from build123d import *

# Parameters (mm, degrees)
SKETCH1_R                = 5.5
SKETCH1_R_2              = 3.9
BOSS_EXTRUDE1_DEPTH      = 14
BOSS_EXTRUDE2_DEPTH      = 30.85
BOSS_EXTRUDE2_DEPTH_BACK = 30.85
SKETCH3_R                = 10
BOSS_EXTRUDE3_DEPTH      = 12.45
SKETCH4_R                = 10
BOSS_EXTRUDE4_DEPTH      = 12.45
CUT_EXTRUDE1_DEPTH       = 3
CUT_EXTRUDE1_DEPTH_BACK  = 3
CUT_EXTRUDE2_DEPTH       = 3
CUT_EXTRUDE2_DEPTH_BACK  = 3


with BuildPart() as part:
    # Sketch1 → Boss-Extrude1 (new body)
    with BuildSketch(Plane(origin=(0, 0, 0), x_dir=(1, 0, 0), z_dir=(0, 1, 0))):
        with BuildLine():
            Line((-18, -44.5), (18, -44.5))
            ThreePointArc((18, -44.5), (24.717514421, -41.717514421), (27.5, -35))
            Line((27.5, -35), (27.5, 35))
            ThreePointArc((27.5, 35), (24.717514421, 41.717514421), (18, 44.5))
            Line((18, 44.5), (-18, 44.5))
            ThreePointArc((-18, 44.5), (-24.717514421, 41.717514421), (-27.5, 35))
            Line((-27.5, 35), (-27.5, -35))
            ThreePointArc((-27.5, -35), (-24.717514421, -41.717514421), (-18, -44.5))
        make_face()
        with Locations((18, 35)):
            Circle(SKETCH1_R, mode=Mode.SUBTRACT)
        with Locations((18, -35)):
            Circle(SKETCH1_R, mode=Mode.SUBTRACT)
        with Locations((0, 35)):
            Circle(SKETCH1_R_2, mode=Mode.SUBTRACT)
        with Locations((0, -35)):
            Circle(SKETCH1_R_2, mode=Mode.SUBTRACT)
        with Locations((-18, 35)):
            Circle(SKETCH1_R, mode=Mode.SUBTRACT)
        with Locations((-18, -35)):
            Circle(SKETCH1_R, mode=Mode.SUBTRACT)
    extrude(amount=BOSS_EXTRUDE1_DEPTH)

    # Sketch2 → Boss-Extrude2 (add, two sides)
    with BuildSketch(Plane.XY) as boss_extrude2_sk:
        Polygon((-28.085675658, 14), (-27.7, 0), (-22.7, 0), (-22.7, 14), align=None)
    extrude(amount=BOSS_EXTRUDE2_DEPTH)
    extrude(boss_extrude2_sk.sketch, amount=-BOSS_EXTRUDE2_DEPTH_BACK)

    # Sketch3 → Boss-Extrude3 (add)
    with BuildSketch(Plane.XY.offset(25)):
        with BuildLine():
            Line((-29.215236642, 55.002986453), (-27.7, 0))
            Line((-27.7, 0), (27.5, 0))
            Line((27.5, 0), (27.5, 16.676103914))
            ThreePointArc((27.5, 16.676103914), (27.466207658, 16.992703195), (27.366353194, 17.295037634))
            Line((27.366353194, 17.295037634), (3.485336194, 70.014582166))
            ThreePointArc((3.485336194, 70.014582166), (-15.37030771, 79.662563606), (-28.994174525, 63.445008121))
            Line((-28.994174525, 63.445008121), (-29.215236642, 55.002986453))
        make_face()
        with Locations((-12, 63)):
            Circle(SKETCH3_R, mode=Mode.SUBTRACT)
    extrude(amount=-BOSS_EXTRUDE3_DEPTH)

    # Sketch4 → Boss-Extrude4 (add)
    with BuildSketch(Plane.XY.offset(-25)):
        with BuildLine():
            Line((-29.215236642, 55.002986453), (-27.7, 0))
            Line((-27.7, 0), (27.5, 0))
            Line((27.5, 0), (27.5, 16.676103914))
            ThreePointArc((27.5, 16.676103914), (27.466207658, 16.992703195), (27.366353194, 17.295037634))
            Line((27.366353194, 17.295037634), (3.485336194, 70.014582166))
            ThreePointArc((3.485336194, 70.014582166), (-15.37030771, 79.662563606), (-28.994174525, 63.445008121))
            Line((-28.994174525, 63.445008121), (-29.215236642, 55.002986453))
        make_face()
        with Locations((-12, 63)):
            Circle(SKETCH4_R, mode=Mode.SUBTRACT)
    extrude(amount=BOSS_EXTRUDE4_DEPTH)

    # Sketch5 → Cut-Extrude1 (cut, two sides)
    with BuildSketch(Plane.XY.offset(25)) as cut_extrude1_sk:
        with BuildLine():
            Line((-9.85, 49.15), (-9.85, 63))
            Line((-9.85, 63), (-14.15, 63))
            Line((-14.15, 63), (-14.15, 49.15))
            ThreePointArc((-14.15, 49.15), (-12, 47), (-9.85, 49.15))
        make_face()
    extrude(amount=CUT_EXTRUDE1_DEPTH, mode=Mode.SUBTRACT)
    extrude(cut_extrude1_sk.sketch, amount=-CUT_EXTRUDE1_DEPTH_BACK, mode=Mode.SUBTRACT)

    # Sketch6 → Cut-Extrude2 (cut, two sides)
    with BuildSketch(Plane.XY.offset(-25)) as cut_extrude2_sk:
        with BuildLine():
            Line((-9.85, 49.15), (-9.85, 63))
            Line((-9.85, 63), (-14.15, 63))
            Line((-14.15, 63), (-14.15, 49.15))
            ThreePointArc((-14.15, 49.15), (-12, 47), (-9.85, 49.15))
        make_face()
    extrude(amount=CUT_EXTRUDE2_DEPTH, mode=Mode.SUBTRACT)
    extrude(cut_extrude2_sk.sketch, amount=-CUT_EXTRUDE2_DEPTH_BACK, mode=Mode.SUBTRACT)


solid = part.part
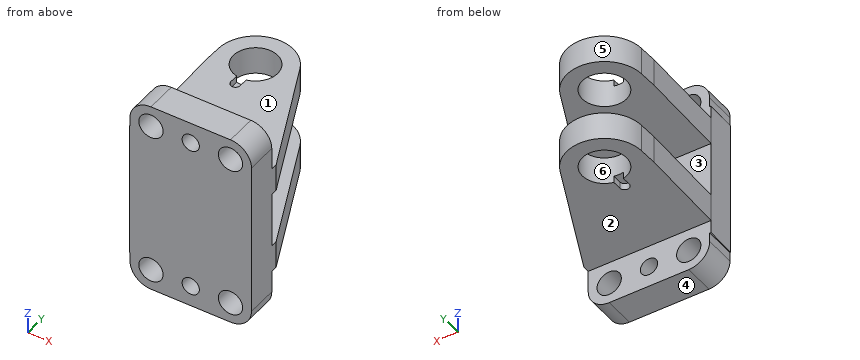
Check sheet for the modelled part. Datum: model origin and axes. Units: mm. Face numbers are marked on the shaded views. A direction names the side the tool comes from. Give positions to 0.01 mm unless a question says otherwise; leave off trailing zeros. Loops run counter-clockwise (first coordinate to the right, second up) from the corner with the lowest first, then second, coordinate; pieces in that order, holes last. Notation, with made-up numbers: M 69.5,25.5 L 94.5,25.5 A18 ccw 94.5,41.5 Z; hole C 82,84 d8. An arc over 180 degrees is marked long. Return JSON: item names as keys, results as strings. Group by question number.
1. Cross-section at C-C on y = 75. Record the boundary of the cut face in (x, z), plus the area to 3 significant figures.
2. Cross-section at B-B on x = 0. Record the boundary of the cut face in (y, z).
3. Cross-section at D-D on z = -8.5. Record the boundary of the cut face in (x, y), plus the area to 4 significant figures.
4. Mould release check, pull along X, two halves, no side actions. Record for the marked faces 4, 5 and 6: released by +X, released by -X, zero draft, split by the parting line, or undercut.
5. Tool access check on the marked faces 1, 2 and 3. Record the directions out of +Z, -Z, +X, -X, +Y, -Y that give a thin tool (end or side, any length) a straight path to the whole face; none if there is none.
6. Thickness scan on L1, parallel to X at y = 5, z = 35; L2, parallel to Z at x = 18, y = 3; L3, parallel to Z at x = 0, y = 10. Record the ranges inside material, lowest first.
7. Go/stop test with flat-tipped pins: pin 1 (3 mm diameter, centred on y = 43.5, z = 23, fed in from -X); pin 2 (4.5 mm diameter, centred on x = -12, y = 51, fed in from -Z); pin 3 (3 mm diameter, centred on y = 62.5, z = -26, fed in from +X); pin 4 (12.5 mm diameter, centred on x = -18, z = 35, fed in from -Y). Record where each tip stops, or that it passes through.
8. Cross-section at A-A on y = 66.5. Record the boundary of the cut face in (x, z).
Return value:
{
 "1": {"outline": "M -24.04,-25 L 0.04,-25 L 0.04,-12.55 L -24.04,-12.55 Z; M -24.04,12.55 L 0.04,12.55 L 0.04,25 L -24.04,25 Z", "area": "600 mm^2"},
 "2": {"outline": "M 0,-44.5 L 14,-44.5 L 14,-38.9 L 0,-38.9 Z; M 0,-31.1 L 14,-31.1 L 14,-25 L 75.04,-25 L 75.04,-12.55 L 14,-12.55 L 14,12.55 L 75.04,12.55 L 75.04,25 L 14,25 L 14,31.1 L 0,31.1 Z; M 0,38.9 L 14,38.9 L 14,44.5 L 0,44.5 Z"},
 "3": {"outline": "M -28.09,14 L -27.7,0 L 27.5,0 L 27.5,14 Z", "area": "775.5 mm^2"},
 "4": {"face 4": "zero draft", "face 5": "split by the parting line", "face 6": "undercut"},
 "5": {"face 1": "+Z, +X, -X, +Y", "face 2": "-Z, +X, -X, +Y", "face 3": "+X, -X, +Y"},
 "6": {"L1": "-27.5 to -23.5, -12.5 to -3.9, 3.9 to 12.5, 23.5 to 27.5", "L2": "-44.5 to -40.5, -29.5 to 29.5, 40.5 to 44.5", "L3": "-44.5 to -38.9, -31.1 to 31.1, 38.9 to 44.5"},
 "7": {"pin 1": "x = -28.94", "pin 2": "z = -25", "pin 3": "x = 7.4", "pin 4": "y = 0"},
 "8": {"outline": "M -28.64,-25 L -21.37,-25 L -21.37,-12.55 L -28.64,-12.55 Z; M -28.64,12.55 L -21.37,12.55 L -21.37,25 L -28.64,25 Z; M -2.63,-25 L 5.08,-25 L 5.08,-12.55 L -2.63,-12.55 Z; M -2.63,12.55 L 5.08,12.55 L 5.08,25 L -2.63,25 Z"}
}
